Read the model definition and answer for the solid it produces. Units are mm, in the model's axes. A direction names the side the tool comes from. Give positions to 0.01 mm unless a question says otherwise; leave off trailing zeros. Write each loop counter-clockwise with the first axis right and the second up, starting at its lowest first coordinate (ties: lowest second). Pieces come first, ordered by that corner, then holes. Notation, with made-up numbers: (88.25, 54.25) -> (143.25, 54.25) arc R31 cw to (143.25, 92.25) -> close; hole circle Ø5 at (-30, 43). An arc over 180 degrees is marked (long way). Answer as CSV lines item,"result". Start each with the question number.
1. For a pull along Z with two mould halves and no side action, classify faces 4 (the flat face through (3, -41, 2.444)), 5 (the flat face through (3, -41, -7.716)), 6 (the flat face through (3, 19.164, 10)), 7 (the flat face through (3, 17, -22.956)) as pulls with the +Z half, pulls with the -Z half, needs draft (parallel to the pull), parting line crosses it, or undercut.
2. A tool of negligible diameter and unlimited length cuts with its end or side. For faces 1 (the flat face through (3, -41, 7.524)), 2 (the flat face through (3, 14.084, 5)), 3 (the flat face through (3, 14.084, -27)), from which of +Z, -Z, +X, -X, +Y, -Y can it reach the whole face along a straight path? Write none if from no direction.
3. The part is cut by section A-A, the plane z = 14.5. Determine the outline of the cut face in (x, y).
4. Find the intervals of material crossed by line 1 (Z direction, x = 2.95, y = -39.5); line 2 (Y direction, x = 3.9, z = -17), in increasing order.
5. Given pin 1 (2.5 mm diameter, centred on x = 2, y = -40, fed in from -Z); pin 2 (2 mm diameter, centred on y = -15.5, z = 7.5, fed in from -X); pin 3 (2.5 mm diameter, centred on x = 1.5, z = 15, fed in from -Y); pin 4 (2.5 mm diameter, centred on x = 1.5, z = -27.5, fed in from +Y), each flat-ended and moving along its own axis, determine where each tip first touches the part or whether it passes through.
from build123d import *

# Parameters (mm, degrees)
SKETCH1_W           = 50.8
SKETCH1_H           = 52.62626
BOSS_EXTRUDE1_DEPTH = 5.08
SKETCH2_W           = 5.08
SKETCH2_H           = 5.08
BOSS_EXTRUDE2_DEPTH = 5.08


with BuildPart() as part:
    # Sketch1 → Boss-Extrude1 (new body)
    with BuildSketch(Plane(origin=(0, 0, 0), x_dir=(0, 0, -1), z_dir=(1, 0, 0))):
        with Locations((5.176303318, -12.22876981)):
            Rectangle(SKETCH1_W, SKETCH1_H)
    extrude(amount=BOSS_EXTRUDE1_DEPTH)

    # Sketch2 → Boss-Extrude2 (add)
    with BuildSketch(Plane(origin=(5.08, 0, 0), x_dir=(0, 0, -1), z_dir=(1, 0, 0))):
        with Locations((-10.063696682, 16.62436019)):
            Rectangle(SKETCH2_W, SKETCH2_H)
        with Locations((10.256303318, 16.62436019)):
            Rectangle(SKETCH2_W, SKETCH2_H)
        with Locations((20.416303318, 16.62436019)):
            Rectangle(SKETCH2_W, SKETCH2_H)
        with Locations((0.096303318, 16.62436019)):
            Rectangle(SKETCH2_W, SKETCH2_H)
        with Locations((0.096303318, -41.08189981)):
            Rectangle(SKETCH2_W, SKETCH2_H)
        with Locations((-10.063696682, -41.08189981)):
            Rectangle(SKETCH2_W, SKETCH2_H)
        with Locations((20.416303318, -41.08189981)):
            Rectangle(SKETCH2_W, SKETCH2_H)
        with Locations((10.256303318, -41.08189981)):
            Rectangle(SKETCH2_W, SKETCH2_H)
    extrude(amount=-BOSS_EXTRUDE2_DEPTH)


solid = part.part
Results found:
1,face 4,"undercut"
1,face 5,"undercut"
1,face 6,"needs draft"
1,face 7,"pulls with the -Z half"
2,face 1,"+X, -X, -Y"
2,face 2,"+X, -X, +Y"
2,face 3,"-Z, +X, -X, +Y"
3,outline,"(0, -38.54) -> (5.08, -38.54) -> (5.08, 14.08) -> (0, 14.08) -> close"
4,line 1,"z = -22.96 to -17.88, -12.8 to -7.72, -2.64 to 2.44, 7.52 to 12.6"
4,line 2,"y = -38.54 to 14.08"
5,pin 1,"stops at z = -22.96"
5,pin 2,"stops at x = 0"
5,pin 3,"stops at y = -38.54"
5,pin 4,"stops at y = 14.08"
